```python
from build123d import *

# Parameters (mm, degrees)
SKETCH1_W           = 212.725
SKETCH1_H           = 314.325
SKETCH1_W_2         = 177.8
SKETCH1_H_2         = 279.4
BOSS_EXTRUDE1_DEPTH = 139.7
SKETCH4_W           = 9.525
SKETCH4_H           = 4.7625
SKETCH6_W           = 196.85
SKETCH6_H           = 298.45
SKETCH6_W_2         = 177.8
SKETCH6_H_2         = 279.4
CUT_EXTRUDE3_DEPTH  = 6.858


with BuildPart() as part:
    # Sketch1 → Boss-Extrude1 (new body)
    with BuildSketch(Plane.XY):
        Rectangle(SKETCH1_W, SKETCH1_H)
        Rectangle(SKETCH1_W_2, SKETCH1_H_2, mode=Mode.SUBTRACT)
    extrude(amount=-BOSS_EXTRUDE1_DEPTH)

    # Cut-Sweep2: sweep along a path in Sketch5
    with BuildLine(Plane(origin=(0, 0, -139.7), x_dir=(-1, 0, 0), z_dir=(0, 0, -1))) as cut_sweep2_path:
        Line((-88.9, -139.7), (-88.9, 139.7))
        Line((-88.9, 139.7), (88.9, 139.7))
        Line((88.9, 139.7), (88.9, -139.7))
        Line((88.9, -139.7), (-88.9, -139.7))
    # Sketch4 → Cut-Sweep2 (sweep, cut)
    with BuildSketch(Plane(origin=(0, 0, 0), x_dir=(1, 0, 0), z_dir=(0, 1, 0))):
        with Locations((-93.6625, 131.7625)):
            Rectangle(SKETCH4_W, SKETCH4_H)
    sweep(path=cut_sweep2_path.line, transition=Transition.RIGHT, mode=Mode.SUBTRACT)

    # Sketch6 → Cut-Extrude3 (cut)
    with BuildSketch(Plane.XY):
        Rectangle(SKETCH6_W, SKETCH6_H)
        Rectangle(SKETCH6_W_2, SKETCH6_H_2, mode=Mode.SUBTRACT)
    extrude(amount=-CUT_EXTRUDE3_DEPTH, mode=Mode.SUBTRACT)


solid = part.part
```
Check sheet for the modelled part. Datum: model origin and axes. Units: mm. A direction names the side the tool comes from. Coordinates: 2 decimals unless noted, no trailing zeros. Loops run counter-clockwise (first coordinate to the right, second up) from the corner with the lowest first, then second, coordinate; pieces in that order, holes last.
1) Sectioned sample at A-A (z = -117). Record the boundary of the cut face in (x, y).
2) Sectioned sample at C-C (x = -47). Record the boundary of the cut face in (y, z) (1 decimal).
3) Access from +Z, -Z, +X, -X, +Y, -Y to the whole of each face (thin tool, end or side, straight path). Record for faces 4 (the face through (-103, 1, 0)), 5 (the face through (-1, -157.162, -69)), 6 (the face through (98.425, -2, -3)), 7 (the face through (-94, -12, -129.381)), 8 (the face through (-88.9, -2, -67)).
4) Sectioned sample at B-B (y = -102.5). Record the boundary of the cut face in (x, z) (1 decimal).
5) Material ranges on probe 1 along Y at (x, z) = (-15.5, -60); probe 2 along Y at (x, z) = (-63.5, -131) (1 decimal); probe 3 along X at (y, z) = (51.5, -24), recorded low to high.
6) Release check for a two-part mould opening along X. For faces 1 (the face through (106.362, -2, -69)), 2 (the face through (-95, 12, -139.7)), 3 (the face through (-1, -149.225, -3)) record: released by +X, released by -X, zero draft, split by the parting line, or undercut.
Check sheet entries:
1. outline: (-106.36, -157.16) - (106.36, -157.16) - (106.36, 157.16) - (-106.36, 157.16) - close; hole (-88.9, -139.7) - (88.9, -139.7) - (88.9, 139.7) - (-88.9, 139.7) - close
2. outline: (-157.2, -139.7) - (-139.7, -139.7) - (-139.7, -134.1) - (-149.2, -134.1) - (-149.2, -129.4) - (-139.7, -129.4) - (-139.7, -6.9) - (-149.2, -6.9) - (-149.2, 0) - (-157.2, 0) - close; (139.7, -139.7) - (157.2, -139.7) - (157.2, 0) - (149.2, 0) - (149.2, -6.9) - (139.7, -6.9) - (139.7, -129.4) - (149.2, -129.4) - (149.2, -134.1) - (139.7, -134.1) - close
3. face 4: +Z, +X, -X, +Y, -Y
3. face 5: +Z, -Z, +X, -X, -Y
3. face 6: +Z
3. face 7: none
3. face 8: +Z, -Z
4. outline: (-106.4, -139.7) - (-88.9, -139.7) - (-88.9, -134.1) - (-98.4, -134.1) - (-98.4, -129.4) - (-88.9, -129.4) - (-88.9, -6.9) - (-98.4, -6.9) - (-98.4, 0) - (-106.4, 0) - close; (88.9, -139.7) - (106.4, -139.7) - (106.4, 0) - (98.4, 0) - (98.4, -6.9) - (88.9, -6.9) - (88.9, -129.4) - (98.4, -129.4) - (98.4, -134.1) - (88.9, -134.1) - close
5. probe 1: y = -157.16 to -139.7, 139.7 to 157.16
5. probe 2: y = -157.2 to -149.2, 149.2 to 157.2
5. probe 3: x = -106.36 to -88.9, 88.9 to 106.36
6. face 1: released by +X
6. face 2: zero draft
6. face 3: undercut
